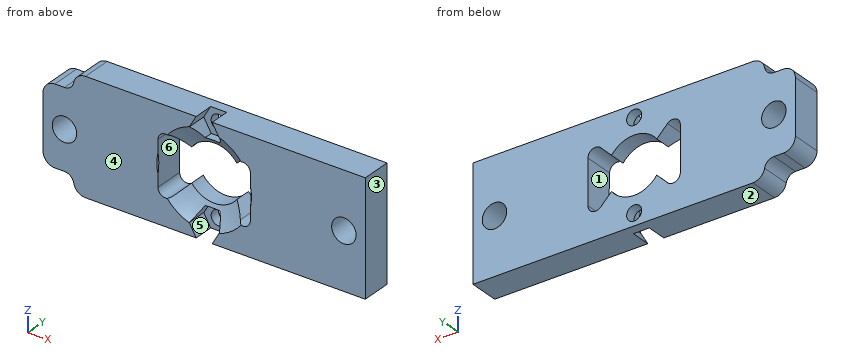
from build123d import *

# Parameters (mm, degrees)
SKETCH2_W           = 68.58
SKETCH2_H           = 24.13
SKETCH2_R           = 2.6
BOSS_EXTRUDE1_DEPTH = 6.35
CUT_EXTRUDE1_DEPTH  = 7.35
FILLET3_R           = 2.54
SKETCH4_R           = 6
CUT_EXTRUDE2_DEPTH  = 7.3500001
SKETCH9_R           = 1.6
CUT_EXTRUDE3_DEPTH  = 7.3500001
CUT_EXTRUDE4_DEPTH  = 4.25


with BuildPart() as part:
    # Sketch2 → Boss-Extrude1 (new body)
    with BuildSketch(Plane(origin=(0, 0, 0), x_dir=(1, 0, 0), z_dir=(0, 1, 0))):
        with Locations((34.29, 12.065)):
            Rectangle(SKETCH2_W, SKETCH2_H)
        with Locations((4.57, 12.065)):
            Circle(SKETCH2_R, mode=Mode.SUBTRACT)
        with Locations((64.01, 12.065)):
            Circle(SKETCH2_R, mode=Mode.SUBTRACT)
    extrude(amount=BOSS_EXTRUDE1_DEPTH)

    # Sketch3 → Cut-Extrude1 (cut, through all)
    with BuildSketch(Plane(origin=(0, 6.35, 0), x_dir=(1, 0, 0), z_dir=(0, 1, 0))):
        with BuildLine():
            Line((4.57, 3.715), (0, 3.715))
            Line((0, 3.715), (0, 0))
            Line((0, 0), (6.57, 0))
            Line((6.57, 0), (6.57, 1.715))
            ThreePointArc((6.57, 1.715), (5.984213562, 3.129213562), (4.57, 3.715))
        make_face()
        with BuildLine():
            ThreePointArc((4.57, 20.415), (5.984213562, 21.000786438), (6.57, 22.415))
            Line((6.57, 22.415), (6.57, 24.13))
            Line((6.57, 24.13), (0, 24.13))
            Line((0, 24.13), (0, 20.415))
            Line((0, 20.415), (4.57, 20.415))
        make_face()
    extrude(amount=-CUT_EXTRUDE1_DEPTH, mode=Mode.SUBTRACT)

    # Fillet3
    fillet3_edges = [part.edges().sort_by_distance(p)[0] for p in [
        (6.57, 3.175, 0),
        (0, 3.175, -3.715),
        (0, 3.175, -20.415),
        (6.57, 3.175, -24.13),
    ]]
    fillet(fillet3_edges, radius=FILLET3_R)

    # Sketch4 → Cut-Extrude2 (cut, through all)
    with BuildSketch(Plane(origin=(0, 6.35, 0), x_dir=(1, 0, 0), z_dir=(0, 1, 0))):
        with Locations((34.29, 12.065)):
            Circle(SKETCH4_R)
    extrude(amount=-CUT_EXTRUDE2_DEPTH, mode=Mode.SUBTRACT)

    # Sketch8 one side → Cut-Revolve6 (revolve, cut)
    with BuildSketch(Plane(origin=(34.29, 0, 0), x_dir=(0, 0, -1), z_dir=(1, 0, 0))):
        with BuildLine():
            Line((12.065, 0), (22.13, 0))
            ThreePointArc((22.13, 0), (17.5473974, 3.215969501), (12.065, 4.35))
            Line((12.065, 4.35), (12.065, 0))
        make_face()
    revolve(axis=Axis((34.29, 6.35, -12.065), (0, -1, 0)), mode=Mode.SUBTRACT)

    # Sketch9 → Cut-Extrude3 (cut, through all)
    with BuildSketch(Plane(origin=(0, 6.35, 0), x_dir=(1, 0, 0), z_dir=(0, 1, 0))):
        with Locations((34.29, 2.565)):
            Circle(SKETCH9_R)
        with Locations((34.29, 21.565)):
            Circle(SKETCH9_R)
        with BuildLine():
            Line((24.462758664, 7.315), (24.462758664, 16.815))
            ThreePointArc((24.462758664, 16.815), (25.450465172, 18.293207252), (27.194129514, 17.94637085))
            Line((27.194129514, 17.94637085), (29.483792257, 15.656708107))
            Line((29.483792257, 15.656708107), (29.483792257, 8.473291893))
            Line((29.483792257, 8.473291893), (27.194129514, 6.18362915))
            ThreePointArc((27.194129514, 6.18362915), (25.450465172, 5.836792748), (24.462758664, 7.315))
        make_face()
        with BuildLine():
            Line((44.117241336, 16.815), (44.117241336, 7.315))
            ThreePointArc((44.117241336, 7.315), (43.129534828, 5.836792748), (41.385870486, 6.18362915))
            Line((41.385870486, 6.18362915), (39.096207743, 8.473291893))
            Line((39.096207743, 8.473291893), (39.096207743, 15.656708107))
            Line((39.096207743, 15.656708107), (41.385870486, 17.94637085))
            ThreePointArc((41.385870486, 17.94637085), (43.129534828, 18.293207252), (44.117241336, 16.815))
        make_face()
    extrude(amount=-CUT_EXTRUDE3_DEPTH, mode=Mode.SUBTRACT)

    # Sketch10 → Cut-Extrude4 (cut)
    with BuildSketch(Plane.XZ):
        Polygon((31.114573519, -21.565), (32.70228676, -24.315), (35.87771324, -24.315), (37.465426481, -21.565), (35.87771324, -18.815), (32.70228676, -18.815), align=None)
        Polygon((32.70228676, -5.315), (35.87771324, -5.315), (37.465426481, -2.565), (35.87771324, 0.185), (32.70228676, 0.185), (31.114573519, -2.565), align=None)
    extrude(amount=-CUT_EXTRUDE4_DEPTH, mode=Mode.SUBTRACT)


solid = part.part
Can you work these out from the model? Positions are in its coordinate system, mm. Face numbers are marked on the shaded views. A direction names the side the tool comes from. Round coordinates to 2 decimals unless told otherwise and drop trailing zeros. Write each loop counter-clockwise with the first axis right and the second up, starting at its lowest first coordinate (ties: lowest second). Pieces come first, ordered by that corner, then holes. Notation, with made-up numbers: (57, -17.5) -> (84, -17.5) arc R5 ccw to (84, -11.5) -> close; hole circle Ø1 at (35, -18). An arc over 180 degrees is marked (long way). One line per question, with ' | ' between items. Start each with the question number.
1) I need wall thicknesses on line 1 (Z direction, x = 34.29, y = 5.2) (3 decimals); line 2 (X direction, y = 1, z = -13.5); line 3 (X direction, y = 1.5, z = -8.75). Which ranges of each line are inside material? Lowest first, please. Write a range as [from, to].
2) If we mould it in two halves opening along Z, with no side actions, what happens to the marked faces 1, 2 and 3? For each: released by +Z, released by -Z, zero draft, split by the parting line, or undercut.
3) Suppose I cut it at B-B on x = 34.29. Count the separate pieces of the cut face and the enclosed holes in it, then the cut area to 3 significant figures.
4) On a 3-axis mill with a long thin cutter (end or side, diameter ignored), from which of +Z, -Z, +X, -X, +Y, -Y can I reach the whole of each face in a straight line? I mean the marked faces 4, 5 and 6. Say none if no direction works.
5) I'm going to push flat-ended pins straight in: P1, Ø2.5, axis at x = 34.5, z = -2, coming from the -Y side; P2, Ø0.9, axis at x = 34.5, y = 3.5, coming from the -Z side (3 decimals); P3, Ø0.5, axis at x = 34, y = 3.5, coming from the +Z side (3 decimals). Where does each tip first touch, or does it pass through?
6) Suppose I cut it at A-A on x = 64.01. Write out the boundary of the cut face in (y, z) (3 decimals), then the cut area to 3 significant figures.
Return value:
1) line 1: z = [-24.13, -23.165], [-19.965, -18.065], [-6.065, -4.165], [-0.965, 0] | line 2: x = [0, 2.4], [6.74, 24.46], [44.12, 61.84], [66.18, 68.58] | line 3: x = [0, 24.46], [44.12, 68.58]
2) face 1: undercut | face 2: released by -Z | face 3: zero draft
3) separate pieces: 4 | enclosed holes: 0 | area: 14.2 mm2
4) face 4: +Z, -Z, +X, -X, -Y | face 5: -Y | face 6: +Y, -Y
5) P1: stops at y = 4.25 | P2: stops at z = -18.815 | P3: stops at z = -5.315
6) outline: (0, -24.13) -> (6.35, -24.13) -> (6.35, -14.665) -> (0, -14.665) -> close; (0, -9.465) -> (6.35, -9.465) -> (6.35, 0) -> (0, 0) -> close | area: 120 mm2
